Source: CAD feature listing. Evaluate the final solid. Frame: model axes, mm. A direction names the side the tool comes from. Round coordinates to 2 decimals unless told otherwise and drop trailing zeros. Order: outer loops, then holes, each group sorted by start corner. A loop starts at its lowest first (then second) coordinate and runs counter-clockwise, first axis right, second up. Notation, with made-up numbers: (26.25, -9.5) - (72.25, -9.5) arc R22 cw to (72.25, 11.5) - close; hole circle Ø6 at (29, -11.75). An arc over 180 degrees is marked (long way). Put each result on its own line as item: value. Start each with the question number.
1) Line query: probe 1 along Y at (x, z) = (389.5, 1.5); probe 2 along X at (y, z) = (-4, 0); probe 3 along X at (y, z) = (-3, -7). Output: solid intervals per line, ascending. Write a range as [from, to].
2) Mould query, pull axis Y, two halves, no side actions, for faces 1 (the face through (670, -55, 0)), 2 (the face through (-54.987, -1.209, -0.245)), 3 (the face through (-39.99, -0.88, 0.25)). Classes: +Y half, -Y half, draft (parallel to the pull), parting line (faces both ways), or undercut.
3) Section B-B on x = 625. Output: boundary loops of the cut face in (y, z).
4) Access query for faces 4 (the face through (670, -40, 0)), 5 (the face through (690, 55, 0)). Directions: +Z, -Z, +X, -X, +Y, -Y. A direction counts if a zero-diameter tool reaches every point of the face in a straight line with its end or side. Return the directions, or none.
5) Section C-C on z = 1. Output: boundary loops of the cut face in (x, y), then the cut area to 3 significant figures.
6) Contact query for flat-ended pins moving along their axis: P1, Ø1.5, axis at y = 27, z = -12.5, coming from the +X side; P2, Ø12, axis at y = 6.5, z = 5, coming from the -X side; P3, Ø6, axis at y = -38, z = 4.5, coming from the +X side. Output: stop coordinate, or through.
7) Section A-A on y = 0. Output: boundary loops of the cut face in (x, z), then the cut area to 3 significant figures.
```python
from build123d import *


with BuildPart() as part:
    # Austragung1: sweep along a path in Skizze2
    with BuildLine(Plane.XY) as austragung1_path:
        Line((0, 40), (1360, 40))
        ThreePointArc((1360, 40), (1400, 0), (1360, -40))
        Line((1360, -40), (0, -40))
        ThreePointArc((0, -40), (-40, 0), (0, 40))
    # 3D-Skizze1 → Austragung1 (sweep)
    with BuildSketch(Plane(origin=(1360, 55, -17.5), x_dir=(0, -0.39391929857916763, 0.9191450300180579), z_dir=(-1, 0, 0))):
        Polygon((0, 0), (32.170076051, 13.78717545), (38.078865529, 0), (5.908789479, -13.78717545), align=None)
    sweep(path=austragung1_path.line)


solid = part.part
```
Answer sheet:
1. probe 1: [-55, -40], [40, 55]
1. probe 2: [-54.85, -39.8], [1399.8, 1414.85]
1. probe 3: [-54.92, -39.89], [1399.89, 1414.92]
2. face 1: -Y half
2. face 2: parting line
2. face 3: undercut
3. outline: (-55, -17.5) - (-40, -17.5) - (-40, 17.5) - (-55, 17.5) - close; (40, -17.5) - (55, -17.5) - (55, 17.5) - (40, 17.5) - close
4. face 4: +Z, -Z
4. face 5: +Z, -Z, +X, -X, +Y
5. outline: (0, -55) - (1360, -55) arc R55 ccw to (1360, 55) - (0, 55) arc R55 ccw to start; hole (0, -40) - (1360, -40) arc R40 ccw to (1360, 40) - (0, 40) arc R40 ccw to start
5. area: 45,300 mm^2
6. P1: x = 1408.33
6. P2: x = -55
6. P3: x = 1402.43
7. outline: (-55, -17.5) - (-40, -17.5) - (-40, 17.5) - (-55, 17.5) - close; (1400, -17.5) - (1415, -17.5) - (1415, 17.5) - (1400, 17.5) - close
7. area: 1,050 mm^2
